Check sheet for the drawn part. Datum: minimum x, y, z corner. Units: mm. Coordinates: 2 decimals unless noted, no trailing zeros. Loops run counter-clockwise (first coordinate to the right, second up) from the corner with the lowest first, then second, coordinate; pieces in that order, holes last. Notation, with made-up numbers: (77.5, 0) - (98.5, 0) arc R29 cw to (98.5, 26) - close; hole circle Ø5 at (86.25, -17.75). An arc over 180 degrees is marked (long way). Answer as a JSON object with one key per item and string values. Group by question number.
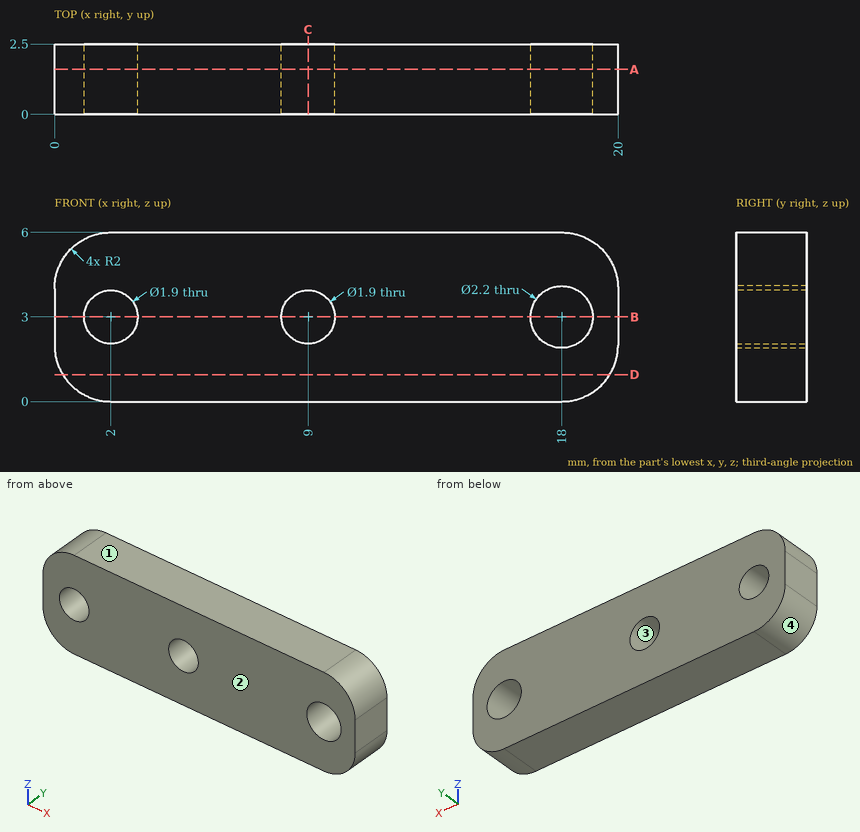
1. Sectioned sample at D-D on z = 0.95. Record the cut outline in (x, y), plus the area to 3 significant figures.
2. Sectioned sample at A-A on y = 1.6. Record the cut outline in (x, z), plus the area to 3 significant figures.
3. Sectioned sample at B-B on z = 3. Record the cut outline in (x, y), plus the area to 3 significant figures.
4. Release check for a two-part mould opening along Z. For the marked faces 1, 2, 3 and 4 record: released by +Z, released by -Z, zero draft, split by the parting line, or undercut.
5. Material ranges on line 1 (X direction, y = 0.75, z = 3); line 2 (Z direction, x = 18, y = 0.6); line 3 (X direction, y = 0.6, z = 2.35), recorded low to high.
6. Gauge pin test, flat end, axial feed: pin 1 (1.3 mm diameter, centred on x = 18, z = 3, fed in from -Y). Record the tip position at first contact, or that the pin passes through.
7. Sectioned sample at C-C on x = 9. Record the cut outline in (y, z).
Answers follow:
{
 "1": {"outline": "(0.3, 0) - (19.7, 0) - (19.7, 2.5) - (0.3, 2.5) - close", "area": "48.5 mm^2"},
 "2": {"outline": "(0, 2) arc R2 ccw to (2, 0) - (18, 0) arc R2 ccw to (20, 2) - (20, 4) arc R2 ccw to (18, 6) - (2, 6) arc R2 ccw to (0, 4) - close; hole circle Ø1.9 at (2, 3); hole circle Ø1.9 at (9, 3); hole circle Ø2.2 at (18, 3)", "area": "107 mm^2"},
 "3": {"outline": "(0, 0) - (1.05, 0) - (1.05, 2.5) - (0, 2.5) - close; (2.95, 0) - (8.05, 0) - (8.05, 2.5) - (2.95, 2.5) - close; (9.95, 0) - (16.9, 0) - (16.9, 2.5) - (9.95, 2.5) - close; (19.1, 0) - (20, 0) - (20, 2.5) - (19.1, 2.5) - close", "area": "35.0 mm^2"},
 "4": {"face 1": "released by +Z", "face 2": "zero draft", "face 3": "undercut", "face 4": "released by -Z"},
 "5": {"line 1": "x = 0 to 1.05, 2.95 to 8.05, 9.95 to 16.9, 19.1 to 20", "line 2": "z = 0 to 1.9, 4.1 to 6", "line 3": "x = 0 to 1.31, 2.69 to 8.31, 9.69 to 17.11, 18.89 to 20"},
 "6": {"pin 1": "passes through"},
 "7": {"outline": "(0, 0) - (2.5, 0) - (2.5, 2.05) - (0, 2.05) - close; (0, 3.95) - (2.5, 3.95) - (2.5, 6) - (0, 6) - close"}
}
